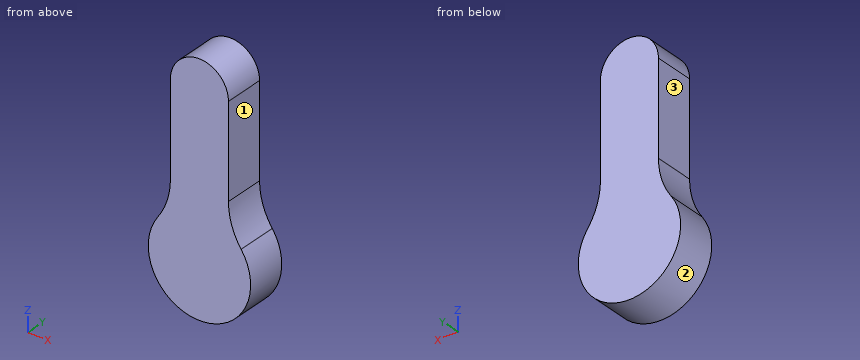
from build123d import *

# Parameters (mm, degrees)
SKETCH1_R           = 7.5
BOSS_EXTRUDE1_DEPTH = 6
FILLET1_R           = 10


with BuildPart() as part:
    # Sketch1 → Boss-Extrude1 (new body)
    with BuildSketch(Plane(origin=(0, 0, 0), x_dir=(1, 0, 0), z_dir=(0, 1, 0))):
        Circle(SKETCH1_R)
        with BuildLine():
            Line((-4.25, 0), (-4.25, -23.75))
            ThreePointArc((-4.25, -23.75), (0, -28), (4.25, -23.75))
            Line((4.25, -23.75), (4.25, 0))
            ThreePointArc((4.25, 0), (0, 4.25), (-4.25, 0))
        make_face()
    extrude(amount=BOSS_EXTRUDE1_DEPTH)

    # Fillet1
    fillet1_edges = [part.edges().sort_by_distance(p)[0] for p in [
        (4.25, 3, 6.179603547),
        (-4.25, 3, 6.179603547),
    ]]
    fillet(fillet1_edges, radius=FILLET1_R)


solid = part.part
Design review of the part built by this model. Coordinates are the model's own, in mm. Face numbers are marked on the shaded views. A direction names the side the tool comes from. Round coordinates to 2 decimals unless told otherwise and drop trailing zeros. Write each loop counter-clockwise with the first axis right and the second up, starting at its lowest first coordinate (ties: lowest second). Pieces come first, ordered by that corner, then holes. Notation, with made-up numbers: (-34.75, 70) -> (-27.75, 70) arc R20 ccw to (-27.75, 103) -> close; hole circle Ø9 at (68, -26). An arc over 180 degrees is marked (long way). One line per item, written item: value. Start each with the question number.
Q1. To check wall thickness, follow probe 1 along X at (y, z) = (1.5, 19.5); probe 2 along Z at (x, y) = (-5.25, 2.4); probe 3 along Z at (x, y) = (-3.5, 5.2). State the ranges of each line that lie inside material, in increasing order.
Q2. Add section B-B (z = 21). Give the boundary of the cut face in (x, y), then the cut area to 3 significant figures.
Q3. Add section C-C (x = 1.75). Give the boundary of the cut face in (y, z).
Q4. Tool access review of the marked faces 1, 2 and 3: name each direction out of +Z, -Z, +X, -X, +Y, -Y from which nothing blocks a thin tool from reaching the whole face with its end or side.
Q5. Add section A-A (y = 4.3). Give the boundary of the cut face in (x, z), then the cut area to 3 significant figures.
Q6. Insertion check: P1, Ø1.5, axis at x = -5, y = 1.5, coming from the -Z side; P2, Ø3, axis at x = -4.5, y = 2, coming from the +Z side; P3, Ø1.8, axis at y = 2.5, z = 17.5, coming from the -X side. Each pin has a flat end and moves straight along its axis. Give the tip position at first contact, or say it passes through.
Response:
1. probe 1: x = -4.25 to 4.25
1. probe 2: z = -5.36 to 5.8
1. probe 3: z = -6.63 to 26.16
2. outline: (-4.25, 0) -> (4.25, 0) -> (4.25, 6) -> (-4.25, 6) -> close
2. area: 51.0 mm^2
3. outline: (0, -7.29) -> (6, -7.29) -> (6, 27.62) -> (0, 27.62) -> close
4. face 1: +Z, +X, +Y, -Y
4. face 2: +Y, -Y
4. face 3: +Z, -X, +Y, -Y
5. outline: (-6.11, 4.35) arc R7.5 ccw (long way) to (6.11, 4.35) arc R10 cw to (4.25, 10.16) -> (4.25, 23.75) arc R4.25 ccw to (-4.25, 23.75) -> (-4.25, 10.16) arc R10 cw to start
5. area: 350 mm^2
6. P1: stops at z = -6.18
6. P2: stops at z = 26.76
6. P3: stops at x = -4.25
